```python
from build123d import *

# Parameters (mm, degrees)
F0_W     = 90
F0_H     = 120
F1_DEPTH = 30
F2_T     = -2.5
F3_R     = 1.5
F4_DEPTH = 25


with BuildPart() as f1:
    # F0 (on Front) → F1 (new body)
    with BuildSketch(Plane.XZ):
        with Locations((-45, 60)):
            Rectangle(F0_W, F0_H)
    extrude(amount=F1_DEPTH)

    # F2
    f2_openings = [f1.faces().sort_by_distance(p)[0] for p in [
        (-45, -30, 60),
    ]]
    offset(amount=F2_T, openings=f2_openings)

    # F3 (on face) → F4 (cut)
    with BuildSketch(Plane.XY.offset(120)):
        with Locations((-45, -15)):
            Circle(F3_R)
    extrude(amount=-F4_DEPTH, mode=Mode.SUBTRACT)


solid = f1.part
```
Source: CAD feature listing. Evaluate the final solid. Frame: model axes, mm. A direction names the side the tool comes from. Give positions to 0.01 mm unless a question says otherwise; leave off trailing zeros. Order: outer loops, then holes, each group sorted by start corner. A loop starts at its lowest first (then second) coordinate and runs counter-clockwise, first axis right, second up.
(1) Material intervals for line 1 along X through (y, z) = (-4.75, 40.5); line 2 along Z through (x, y) = (-72, -16.75); line 3 along Y through (x, z) = (-45, 119.2), sorted ascending.
(2) Section query A-A (x = -45). Return the cut outline in (y, z).
(3) Section query D-D (x = -22.5). Return the cut outline in (y, z).
(4) Access query for faces 4 (the face through (-46, -11, 120)), 5 (the face through (-46.5, -14.93, 118.77)), 6 (the face through (-87.5, -16, 59)). Directions: +Z, -Z, +X, -X, +Y, -Y. A direction counts if a zero-diameter tool reaches every point of the face in a straight line with its end or side. Return the directions, or none.
(5) Pull-direction query (X, two-part tool) for faces 1 (the face through (-45, -30, 118)), 2 (the face through (-90, -15, 59)), 3 (the face through (-46, -13, 117.5)); classes: +X half, -X half, draft (parallel to the pull), parting line (faces both ways), or undercut.
(6) Section query B-B (y = -25.5). Return the cut outline in (x, z), plus the area to 4 significant figures.
(7) Section query C-C (z = 25). Return the cut outline in (x, y).
Outcome:
1. line 1: x = -90 to -87.5, -2.5 to 0
1. line 2: z = 0 to 2.5, 117.5 to 120
1. line 3: y = -30 to -16.5, -13.5 to 0
2. outline: (-30, 0) - (0, 0) - (0, 120) - (-13.5, 120) - (-13.5, 117.5) - (-2.5, 117.5) - (-2.5, 2.5) - (-30, 2.5) - close; (-30, 117.5) - (-16.5, 117.5) - (-16.5, 120) - (-30, 120) - close
3. outline: (-30, 0) - (0, 0) - (0, 120) - (-30, 120) - (-30, 117.5) - (-2.5, 117.5) - (-2.5, 2.5) - (-30, 2.5) - close
4. face 4: +Z, +X, -X, +Y, -Y
4. face 5: +Z
4. face 6: -Y
5. face 1: draft
5. face 2: -X half
5. face 3: undercut
6. outline: (-90, 0) - (0, 0) - (0, 120) - (-90, 120) - close; hole (-87.5, 2.5) - (-2.5, 2.5) - (-2.5, 117.5) - (-87.5, 117.5) - close
6. area: 1,025 mm2
7. outline: (-90, -30) - (-87.5, -30) - (-87.5, -2.5) - (-2.5, -2.5) - (-2.5, -30) - (0, -30) - (0, 0) - (-90, 0) - close
